The model under review builds one solid part; all positions refer to its coordinate system, in mm. A direction names the side the tool comes from. Round coordinates to 2 decimals unless told otherwise and drop trailing zeros. Write each loop counter-clockwise with the first axis right and the second up, starting at its lowest first coordinate (ties: lowest second). Pieces come first, ordered by that corner, then holes. Notation, with made-up numbers: (-4, 71.25) - (38, 71.25) arc R37 ccw to (38, 109.25) - close; hole circle Ø1 at (-11.5, 9.25). An arc over 180 degrees is marked (long way). Return JSON: item names as keys, results as strings.
from build123d import *

# Parameters (mm, degrees)
BOSS_EXTRUDE1_DEPTH = 0.6
SKETCH3_W           = 9
SKETCH3_H           = 16
BOSS_EXTRUDE2_DEPTH = 2.4
SKETCH4_W           = 16
SKETCH4_H           = 20
BOSS_EXTRUDE3_DEPTH = 10
SKETCH5_R           = 5.1
CUT_EXTRUDE1_DEPTH  = 10
SKETCH6_R           = 5.1
CUT_EXTRUDE3_DEPTH  = 10
SKETCH7_R           = 5.1
CUT_EXTRUDE4_DEPTH  = 10
FILLET1_R           = 2
SKETCH8_W           = 2.2
SKETCH8_H           = 2.2
CUT_EXTRUDE5_DEPTH  = 3
SKETCH9_W           = 2.2
SKETCH9_H           = 2.2
CUT_EXTRUDE6_DEPTH  = 3
SKETCH10_W          = 2.2
SKETCH10_H          = 2.2
CUT_EXTRUDE7_DEPTH  = 3


with BuildPart() as part:
    # Sketch2 → Boss-Extrude1 (new body)
    with BuildSketch(Plane(origin=(0, 0, 0), x_dir=(1, 0, 0), z_dir=(0, 1, 0))):
        Polygon((-56, 8), (56, 8), (63, 8), (63, -8), (56, -8), (-56, -8), align=None)
    extrude(amount=-BOSS_EXTRUDE1_DEPTH)

    # Sketch3 → Boss-Extrude2 (add)
    with BuildSketch(Plane(origin=(0, 0, 0), x_dir=(1, 0, 0), z_dir=(0, 1, 0))):
        with Locations((44.5, 0)):
            Rectangle(SKETCH3_W, SKETCH3_H)
        with Locations((18, 0)):
            Rectangle(SKETCH3_W, SKETCH3_H)
        with Locations((-26.5, 0)):
            Rectangle(SKETCH3_W, SKETCH3_H)
    extrude(amount=BOSS_EXTRUDE2_DEPTH)

    # Sketch4 → Boss-Extrude3 (add)
    with BuildSketch(Plane(origin=(0, 2.4, 0), x_dir=(1, 0, 0), z_dir=(0, 1, 0))):
        with Locations((-23, 0)):
            Rectangle(SKETCH4_W, SKETCH4_H)
        with Locations((21.5, 0)):
            Rectangle(SKETCH4_W, SKETCH4_H)
        with Locations((48, 0)):
            Rectangle(SKETCH4_W, SKETCH4_H)
    extrude(amount=BOSS_EXTRUDE3_DEPTH)

    # Sketch5 → Cut-Extrude1 (cut)
    with BuildSketch(Plane(origin=(56, 0, 0), x_dir=(0, 0, -1), z_dir=(1, 0, 0))):
        with Locations((0, 7.4)):
            Circle(SKETCH5_R)
    extrude(amount=-CUT_EXTRUDE1_DEPTH, mode=Mode.SUBTRACT)

    # Sketch6 → Cut-Extrude3 (cut)
    with BuildSketch(Plane(origin=(29.5, 0, 0), x_dir=(0, 0, -1), z_dir=(1, 0, 0))):
        with Locations((0, 7.4)):
            Circle(SKETCH6_R)
    extrude(amount=-CUT_EXTRUDE3_DEPTH, mode=Mode.SUBTRACT)

    # Sketch7 → Cut-Extrude4 (cut)
    with BuildSketch(Plane(origin=(-15, 0, 0), x_dir=(0, 0, -1), z_dir=(1, 0, 0))):
        with Locations((0, 7.4)):
            Circle(SKETCH7_R)
    extrude(amount=-CUT_EXTRUDE4_DEPTH, mode=Mode.SUBTRACT)

    # Fillet1
    fillet1_edges = [part.edges().sort_by_distance(p)[0] for p in [
        (-23, 12.4, 10),
        (-23, 12.4, -10),
        (48, 12.4, 10),
        (48, 12.4, -10),
        (21.5, 12.4, 10),
        (21.5, 12.4, -10),
    ]]
    fillet(fillet1_edges, radius=FILLET1_R)

    # Sketch8 → Cut-Extrude5 (cut)
    with BuildSketch(Plane.ZY.offset(31)):
        with Locations((6, 7.4)):
            Rectangle(SKETCH8_W, SKETCH8_H)
        with Locations((-6, 7.4)):
            Rectangle(SKETCH8_W, SKETCH8_H)
    extrude(amount=-CUT_EXTRUDE5_DEPTH, mode=Mode.SUBTRACT)

    # Sketch9 → Cut-Extrude6 (cut)
    with BuildSketch(Plane(origin=(13.5, 0, -13.5), x_dir=(0, 0, 1), z_dir=(-1, 0, 0))):
        with Locations((19.5, 7.4)):
            Rectangle(SKETCH9_W, SKETCH9_H)
        with Locations((7.5, 7.4)):
            Rectangle(SKETCH9_W, SKETCH9_H)
    extrude(amount=-CUT_EXTRUDE6_DEPTH, mode=Mode.SUBTRACT)

    # Sketch10 → Cut-Extrude7 (cut)
    with BuildSketch(Plane(origin=(40, 0, -40), x_dir=(0, 0, 1), z_dir=(-1, 0, 0))):
        with Locations((46, 7.4)):
            Rectangle(SKETCH10_W, SKETCH10_H)
        with Locations((34, 7.4)):
            Rectangle(SKETCH10_W, SKETCH10_H)
    extrude(amount=-CUT_EXTRUDE7_DEPTH, mode=Mode.SUBTRACT)


solid = part.part
(1) Add section A-A (y = 1). Write out the cut boundary in (x, z).
Filled in:
{"outline": "(-31, -8) - (-22, -8) - (-22, 8) - (-31, 8) - close; (13.5, -8) - (22.5, -8) - (22.5, 8) - (13.5, 8) - close; (40, -8) - (49, -8) - (49, 8) - (40, 8) - close"}
(2) Add section C-C (x = 11). Write out the cut boundary in (y, z), plus the area to 3 significant figures.
Filled in:
{"outline": "(-0.6, -8) - (0, -8) - (0, 8) - (-0.6, 8) - close", "area": "9.60 mm2"}
(3) Add section B-B (z = 0). Write out the cut boundary in (x, y).
Filled in:
{"outline": "(-56, -0.6) - (63, -0.6) - (63, 0) - (49, 0) - (49, 2.3) - (46, 2.3) - (46, 12.4) - (40, 12.4) - (40, 0) - (22.5, 0) - (22.5, 2.3) - (19.5, 2.3) - (19.5, 12.4) - (13.5, 12.4) - (13.5, 0) - (-22, 0) - (-22, 2.3) - (-25, 2.3) - (-25, 12.4) - (-31, 12.4) - (-31, 0) - (-56, 0) - close"}
(4) For faces 4 (the flat face through (25, 2.4, -7)), 5 (the flat face through (-28, 7, -6)), 6 (the flat face through (15, 7, -7.1)), list the 3-axis set-ups (+Z, -Z, +X, -X, +Y, -Y) from which the entire face can be reached by the end or side of a thin tool; tool diameter is ignored.
Filled in:
{"face 4": "-Z", "face 5": "-X", "face 6": "none"}
(5) Add section D-D (y = 7.4). Give the number of separate pieces and of enclosed holes in the cut face, plus the area to 3 significant figures.
Filled in:
{"separate pieces": "3", "enclosed holes": "0", "area": "614 mm2"}
(6) Clearance check with flat-ended pins moving along their axes: pin 1 Ø3 at (y, z) = (3, -1.5) entering from -X; pin 2 Ø1.1 at (y, z) = (7, -6.5) entering from -X. State where each tip first meets the part, or that it passes through.
Filled in:
{"pin 1": "stops at x = -31", "pin 2": "stops at x = -28"}
(7) Wall thickness on line 1 (X direction, y = 4.5, z = 5.5); line 2 (X direction, y = 11, z = -3.5); line 3 (Z direction, x = 49.75, y = 7.4): over which ranges is each line inside the solid? List them lowest first.
Filled in:
{"line 1": "x = -31 to -15, 13.5 to 29.5, 40 to 56", "line 2": "x = -31 to -25, 13.5 to 19.5, 40 to 46", "line 3": "z = -10 to -5.1, 5.1 to 10"}
(8) Mouldability with a two-part tool opening along Z and no side actions: class faces 1 (the flat face through (-23, 6, -10)), 2 (the cylindrical face through (48.11, 11.83, 9.4)), 3 (the cylindrical face through (-19.9, 11.9, 2.4)) as released by +Z, released by -Z, zero draft, split by the parting line, or undercut.
Filled in:
{"face 1": "released by -Z", "face 2": "released by +Z", "face 3": "undercut"}
